Verification items for this drawing (mm, ordinates from the low corner). Give positions to 0.01 mm unless a question says otherwise; leave off trailing zeros. Loops run counter-clockwise (first coordinate to the right, second up) from the corner with the lowest first, then second, coordinate; pieces in that order, holes last. Notation, with made-up numbers: (73, 27.5) -> (115, 27.5) arc R28 cw to (115, 52.5) -> close; hole circle Ø6 at (69, 6.25). An arc over 180 degrees is marked (long way). Write item = value, one per line.
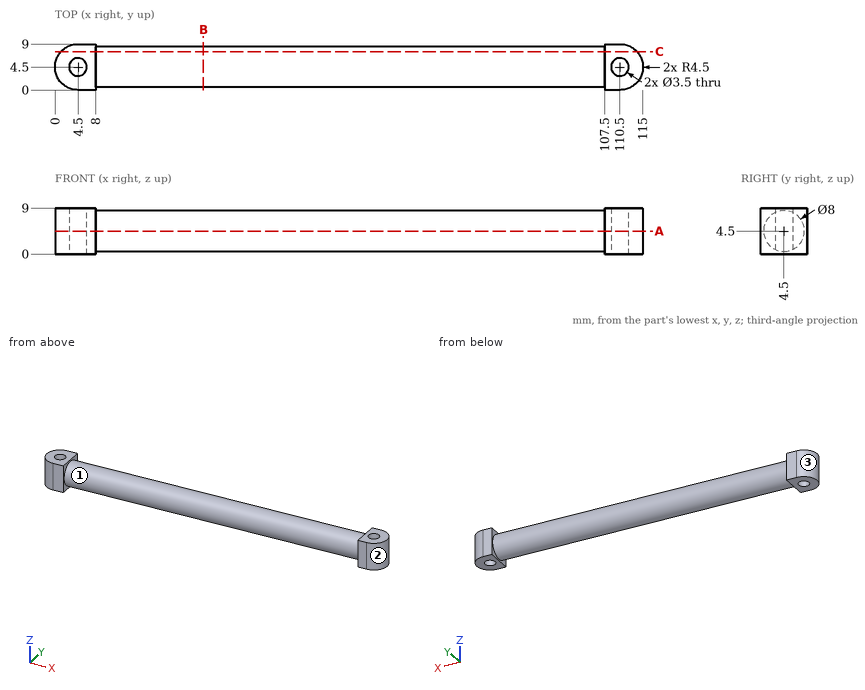
Item 1: Section check A-A, the plane z = 4.5. Record the cut outline in (x, y), plus the area to 3 significant figures.
Answer:
outline = (4.5, 0) -> (8, 0) -> (8, 0.5) -> (107.5, 0.5) -> (107.5, 0) -> (110.5, 0) arc R4.5 ccw to (110.5, 9) -> (107.5, 9) -> (107.5, 8.5) -> (8, 8.5) -> (8, 9) -> (4.5, 9) arc R4.5 ccw to start; hole circle Ø3.5 at (4.5, 4.5); hole circle Ø3.5 at (110.5, 4.5)
area = 899 mm^2
Item 2: Draft check along X on the marked faces 1, 2 and 3. Enter one of: +X half, -X half, draft (parallel to the pull), parting line (faces both ways), or undercut.
Answer:
face_1 = undercut
face_2 = +X half
face_3 = -X half
Item 3: Section check C-C, the plane y = 7.5. Record the cut outline in (x, z), plus the area to 3 significant figures.
Answer:
outline = (1.15, 0) -> (8, 0) -> (8, 1.85) -> (107.5, 1.85) -> (107.5, 0) -> (113.85, 0) -> (113.85, 9) -> (107.5, 9) -> (107.5, 7.15) -> (8, 7.15) -> (8, 9) -> (1.15, 9) -> close
area = 645 mm^2
Item 4: Thickness scan on L1, parallel to Y at x = 110.5, z = 7; L2, parallel to X at y = 3, z = 2; L3, parallel to Y at x = 6, z = 4.5. Record the ranges inside material, lowest first. Write a range as [from, to].
Answer:
L1 = [0, 2.75], [6.25, 9]
L2 = [0.26, 3.6], [5.4, 109.6], [111.4, 114.74]
L3 = [0, 3.6], [5.4, 9]
Item 5: Gauge pin test, flat ends, axial feed: pin 1 (3 mm diameter, centred on y = 6.5, z = 6, fed in from +X); pin 2 (2 mm diameter, centred on x = 56, y = 6, fed in from +Z); pin 3 (5 mm diameter, centred on x = 39, z = 7, fed in from +Y). Record the tip position at first contact, or that the pin passes through.
Answer:
pin_1 = 114.97
pin_2 = 8.47
pin_3 = 8.5
Item 6: Section check B-B, the plane x = 29. Record the cut outline in (y, z).
Answer:
outline = circle Ø8 at (4.5, 4.5)
